Design review of the part built by this model. Coordinates are the model's own, in mm. Face numbers are marked on the shaded views. Coordinates: 2 decimals unless noted, no trailing zeros. Write each loop counter-clockwise with the first axis right and the second up, starting at its lowest first coordinate (ties: lowest second). Pieces come first, ordered by that corner, then holes. Notation, with made-up numbers: (22.5, 61) - (69.5, 61) arc R29 cw to (69.5, 83) - close; hole circle Ø3 at (0, -6). An arc over 180 degrees is marked (long way). Answer as a JSON object with one key per item and string values.
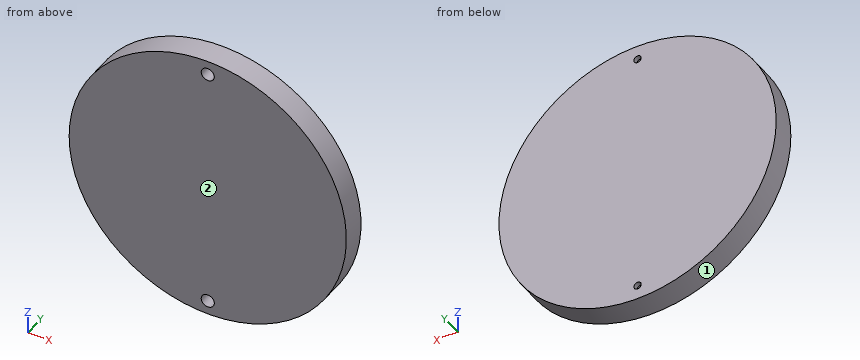
Autodesk Inventor part; units mm, degrees
ref_plane "YZ Plane" through (0, 0, 0) normal (1, 0, 0) x (0, 1, 0)
ref_plane "XZ Plane" through (0, 0, 0) normal (0, 1, 0) x (-1, 0, 0)
ref_plane "XY Plane" through (0, 0, 0) normal (0, 0, 1) x (1, 0, 0)
sketch "Sketch1" plane through (0, 0, 0) normal (0, 1, 0) x (-1, 0, 0)
  circle A0 centre (0, 0) radius 84.75
  dimension "d0" = 169.5
extrude "Extrusion1" add sketch "Sketch1" along normal blind 15
sketch "Sketch2" plane through (0, 0, 0) normal (0, -1, 0) x (1, 0, 0)
  circle A0 centre (0, 0) radius 76
  circle A1 centre (0, 76) radius 4
  circle A2 centre (0, -76) radius 4
  circle A3 centre (0, 76) radius 2.25
  circle A4 centre (0, -76) radius 2.25
  dimension "d3" = 152
  dimension "d4" = 8
  dimension "d5" = 8
  dimension "d6" = 4.5
  dimension "d7" = 4.5
extrude "Extrusion2" cut sketch "Sketch2" against normal through all contours A3 A0 | A0 A3 | A4 A0 | A0 A4
extrude "Extrusion3" cut sketch "Sketch2" against normal blind 12 contours A1 A0 A3 | A0 A3 A1 | A2 A0 A4 | A0 A4 A2 | A3 A0 | A0 A3 | A4 A0 | A0 A4
properties part number "substrate plate"
(1) Take a section at D-D, the plane z = 27. Write out the cut boundary in (x, y).
Solved:
{"outline": "(-80.33, 0) - (80.33, 0) - (80.33, 15) - (-80.33, 15) - close"}
(2) For pin 1 (8 mm diameter, centred on x = -31.5, z = -1, fed in from -Y); pin 2 (7 mm diameter, centred on x = 0, z = -76, fed in from -Y); pin 3 (1.5 mm diameter, centred on x = -65, y = 11, fed in from -Z); pin 4 (1.5 mm diameter, centred on y = 8, z = -18, fed in from +X), all flat-tipped, find the tip position at first contact; note any pin that passes through.
Solved:
{"pin 1": "stops at y = 0", "pin 2": "stops at y = 12", "pin 3": "stops at z = -55.27", "pin 4": "stops at x = 82.98"}
(3) To check wall thickness, follow line 1 (Z direction, x = 0, y = 14.15); line 2 (Z direction, x = 0, y = 9.75); line 3 (X direction, y = 7.5, z = -76). State the ranges of each line that lie inside material, in increasing order. Write a range as from..to.
Solved:
{"line 1": "z = -84.75..-78.25, -73.75..73.75, 78.25..84.75", "line 2": "z = -84.75..-80, -72..72, 80..84.75", "line 3": "x = -37.5..-4, 4..37.5"}
(4) Take a section at B-B, the plane y = 5. Write out the cut boundary in (x, z).
Solved:
{"outline": "circle Ø169.5 at (0, 0); hole circle Ø8 at (0, -76); hole circle Ø8 at (0, 76)"}
(5) Take a section at C-C, the plane x = -54.5. Write out the cut boundary in (y, z).
Solved:
{"outline": "(0, -64.9) - (15, -64.9) - (15, 64.9) - (0, 64.9) - close"}
(6) The part is to be moulded in two halves that separate along X. For the marked faces 1 and 2, say which applies: pulls with the +X half, pulls with the -X half, needs draft (parallel to the pull), parting line crosses it, or undercut.
Solved:
{"face 1": "parting line crosses it", "face 2": "needs draft"}
(7) Take a section at A-A, the plane z = 76. Write out the cut boundary in (x, y), and give its area (3 significant figures).
Solved:
{"outline": "(-37.5, 0) - (-4, 0) - (-4, 12) - (-2.25, 12) - (-2.25, 15) - (-37.5, 15) - close; (2.25, 12) - (4, 12) - (4, 0) - (37.5, 0) - (37.5, 15) - (2.25, 15) - close", "area": "1,020 mm^2"}
